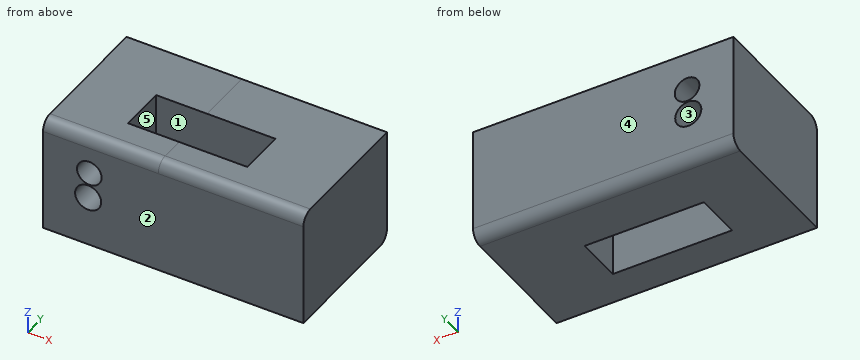
from build123d import *

# Parameters (mm, degrees)
F0_W     = 127
F0_H     = 127
F1_DEPTH = 76.2
F2_R     = 12.7
F3_R     = 13.5576573184
F3_R_2   = 14.3770911371
F4_DEPTH = 152.4
F5_DEPTH = 160.02
F6_W     = 131.4042881131
F6_H     = 51.2029398233
F7_DEPTH = 211.836


with BuildPart() as f1:
    # F0 (on Front) → F1 (new body, symmetric)
    with BuildSketch(Plane.XZ):
        with Locations((63.5, 63.5)):
            Rectangle(F0_W, F0_H)
    extrude(amount=F1_DEPTH, both=True)

    # F2
    f2_edges = [f1.edges().sort_by_distance(p)[0] for p in [
        (63.5, -76.2, 127),
        (63.5, 76.2, 0),
    ]]
    fillet(f2_edges, radius=F2_R)

    # F3 (on face) → F4 (cut, through all)
    with BuildSketch(Plane.XZ.offset(76.2)):
        with Locations((51.0555580258, 84.6957564354)):
            Circle(F3_R)
        with Locations((49.7466027737, 55.3751178086)):
            Circle(F3_R_2)
    extrude(amount=-F4_DEPTH, mode=Mode.SUBTRACT)

    # F5 (add): a face of the model
    f5_faces = [f1.faces().sort_by_distance(p)[0] for p in [
        (127, 0, 63.5),
    ]]
    extrude(f5_faces, amount=F5_DEPTH)

    # F6 (on face) → F7 (cut)
    with BuildSketch(Plane.XY.offset(127)):
        with Locations((136.3636963069, -12.5774694607)):
            Rectangle(F6_W, F6_H)
    extrude(amount=-F7_DEPTH, mode=Mode.SUBTRACT)


solid = f1.part
The model under review builds one solid part; all positions refer to its coordinate system, in mm. Face numbers are marked on the shaded views. A direction names the side the tool comes from. Round coordinates to 2 decimals unless told otherwise and drop trailing zeros. Write each loop counter-clockwise with the first axis right and the second up, starting at its lowest first coordinate (ties: lowest second). Pieces come first, ordered by that corner, then holes. Notation, with made-up numbers: M -3,-35.75 L 49,-35.75 A15 cw 49,-16.75 Z; hole C 36.25,56.5 d5. An arc over 180 degrees is marked long. Answer as CSV lines item,"result". Start each with the question number.
Q1. Consider section D-D, the plane y = -51. Give the boundary of the cut face in (x, z).
Q2. Consider section A-A, the plane z = 52. Give the boundary of the cut face in (x, y), then the cut area to 3 significant figures.
Q3. The part is to be moulded in two halves that separate along Y. For the marked faces 3, 4 and 5, say which applies: +Y half, -Y half, draft (parallel to the pull), parting line (faces both ways), or undercut.
Q4. Consider section C-C, the plane x = 188.5. Give the boundary of the cut face in (y, z).
Q5. Consider section B-B, the plane y = 10. Give the boundary of the cut face in (x, z), then the cut area to 3 significant figures.
Q6. Tool access review of the marked faces 1 and 2: name each direction out of +Z, -Z, +X, -X, +Y, -Y from which nothing blocks a thin tool from reaching the whole face with its end or side.
Q7. Wall thickness on line 1 along Y through (x, z) = (121, 94.5); line 2 along X through (y, z) = (-11.5, 96.5); line 3 along X through (y, z) = (10, 81): over which ranges is each line inside the solid? List them lowest first.
Result set:
1,outline,"M 0,0 L 287.02,0 L 287.02,127 L 0,127 Z; hole C 49.75,55.38 d28.75; hole C 51.06,84.7 d27.12"
2,outline,"M 0,-76.2 L 35.77,-76.2 L 35.77,76.2 L 0,76.2 Z; M 63.72,-76.2 L 287.02,-76.2 L 287.02,76.2 L 63.72,76.2 Z; hole M 70.66,-38.18 L 202.07,-38.18 L 202.07,13.02 L 70.66,13.02 Z"
2,area,"32,800 mm²"
3,face 3,"draft"
3,face 4,"+Y half"
3,face 5,"undercut"
4,outline,"M -76.2,0 L -38.18,0 L -38.18,127 L -63.5,127 A12.7 ccw -76.2,114.3 Z; M 13.02,0 L 63.5,0 A12.7 ccw 76.2,12.7 L 76.2,127 L 13.02,127 Z"
5,outline,"M 0,0 L 70.66,0 L 70.66,127 L 0,127 Z; M 202.07,0 L 287.02,0 L 287.02,127 L 202.07,127 Z; hole C 49.75,55.38 d28.75; hole C 51.06,84.7 d27.12"
5,area,"18,500 mm²"
6,face 1,"+Z, -Z"
6,face 2,"+Z, -Z, +X, -X, -Y"
7,line 1,"y = -76.2 to -38.18, 13.02 to 76.2"
7,line 2,"x = 0 to 44.39, 57.72 to 70.66, 202.07 to 287.02"
7,line 3,"x = 0 to 38.01, 64.1 to 70.66, 202.07 to 287.02"
